The model under review builds one solid part; all positions refer to its coordinate system, in mm. Give positions to 0.01 mm unless a question says otherwise; leave off trailing zeros. Order: outer loops, then holes, each group sorted by start corner. A loop starts at its lowest first (then second) coordinate and runs counter-clockwise, first axis right, second up. Notation, with made-up numbers: M 19.5,26.5 L 62.5,26.5 A16 ccw 62.5,44.5 Z; hole C 17.25,73 d2. An arc over 180 degrees is marked long. One line per question, with ' | ' between items. Start each with the question number.
1. We need section A-A on z = 119. Write out the cut boundary in (x, y), then the cut area to 3 significant figures.
2. Insertion check: P1, Ø2.5, axis at x = 0, z = 342.4, coming from the -Y side; P2, Ø9, axis at x = 0, z = 342.4, coming from the -Y side; P3, Ø9, axis at x = 0, z = 190, coming from the +Y side. Each pin has a flat end and moves straight along its axis. Give the tip position at first contact, or say it passes through.
3. We need section B-B on y = -3.75. Write out the cut boundary in (x, z).
4. Wall thickness on L1, parallel to Y at x = 3.25, z = 20; L2, parallel to X at y = 7.2, z = 240.8: over which ranges is each line inside the solid? List them lowest first.
Autodesk Inventor part; units mm, degrees
ref_plane "YZ Plane" through (0, 0, 0) normal (1, 0, 0) x (0, 1, 0)
ref_plane "XZ Plane" through (0, 0, 0) normal (0, 1, 0) x (-1, 0, 0)
ref_plane "XY Plane" through (0, 0, 0) normal (0, 0, 1) x (1, 0, 0)
sketch "Náčrt1" plane through (0, 0, 0) normal (0, 0, 1) x (1, 0, 0)
  line L0 (-7.5, -7.5) -> (7.5, -7.5)
  line L1 (7.5, -7.5) -> (7.5, 7.5)
  line L2 (7.5, 7.5) -> (-7.5, 7.5)
  line L3 (-7.5, 7.5) -> (-7.5, -7.5)
  line L4 (-7.5, -7.5) -> (7.5, 7.5) construction
  line L5 (7.5, -7.5) -> (-7.5, 7.5) construction
  line L6 (-6.5, -6.5) -> (6.5, -6.5)
  line L7 (6.5, -6.5) -> (6.5, 6.5)
  line L8 (6.5, 6.5) -> (-6.5, 6.5)
  line L9 (-6.5, 6.5) -> (-6.5, -6.5)
  line L10 (-6.5, -6.5) -> (6.5, 6.5) construction
  line L11 (6.5, -6.5) -> (-6.5, 6.5) construction
  point P0 (0, 0)
  dimension "d0" = 15
  dimension "d1" = 15
  dimension "d2" = 13
  dimension "d3" = 13
extrude "Vysunutí1" add sketch "Náčrt1" along normal blind 380
sketch "Náčrt2" plane through (-7.5, 7.5, 0) normal (0, 1, 0) x (1, 0, 0)
  circle A0 centre (7.5, -37.6) radius 1.5
  line L0 (15, 0) -> (0, 0)
  line L1 (0, 0) -> (0, -380)
  line L2 (15, -380) -> (0, -380)
  line L3 (15, 0) -> (15, -380)
  point P0 (7.5, 0)
  dimension "d8" = 3
  dimension "d13" = 37.6
  dimension "d19" = 7.5
extrude "Vysunutí2" cut sketch "Náčrt2" against normal up to surface (1 mm away) contours A0
sketch "Náčrt3" plane through (-7.5, -7.5, 0) normal (0, -1, 0) x (1, 0, 0)
  line L0 (15, 0) -> (0, 0)
  line L1 (0, 0) -> (0, 380)
  line L2 (15, 380) -> (0, 380)
  line L3 (15, 0) -> (15, 380)
  circle A0 centre (7.5, 37.6) radius 1.5
  circle A1 centre (7.5, 37.6) radius 5
  point P0 (7.5, 0)
  dimension "d15" = 10
extrude "Vysunutí3" cut sketch "Náčrt3" against normal up to surface (1 mm away) contours A0 | A1
pattern_linear "Obdélníkové pole1" count 7 spacing 50.8 along (0, 0, 1) of "Vysunutí2"
pattern_linear "Obdélníkové pole2" count 7 spacing 50.8 along (0, 0, 1) of "Vysunutí3"
equation "\"d0\" = width"
equation "\"d1\" = width"
equation "\"d2\" = width - 2 * thickness"
equation "\"d3\" = width - 2 * thickness"
equation "\"d4\" = length"
equation "\"d8\" = HoleDia"
equation "\"d19\" = 0.5 * width"
equation "\"d15\" = HoleDiaOpposite"
equation "\"d22\" = holeDistance"
equation "\"d25\" = holeDistance"
equation "\"width\" = gSquareProfile_Width_Cabinet"
equation "\"thickness\" = gSquareProfile_Thickness_Cabinet"
equation "\"length\" = gCabinet_LogicCircuit_Length - 2 * width"
equation "\"holeDistance\" = 50.8"
equation "\"HoleDiaOpposite\" = 10"
equation "\"HoleDia\" = 3"
properties part number "Profile-Square#07"
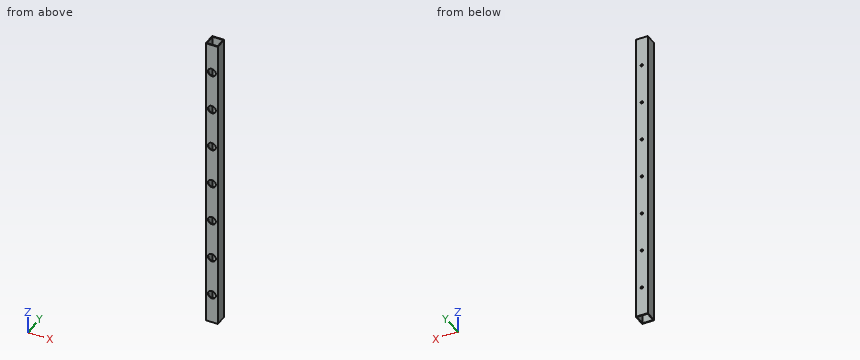
Entries:
1) outline: M -7.5,-7.5 L 7.5,-7.5 L 7.5,7.5 L -7.5,7.5 Z; hole M -6.5,-6.5 L 6.5,-6.5 L 6.5,6.5 L -6.5,6.5 Z | area: 56.0 mm^2
2) P1: passes through | P2: stops at y = 6.5 | P3: stops at y = 7.5
3) outline: M -7.5,0 L -6.5,0 L -6.5,380 L -7.5,380 Z; M 6.5,0 L 7.5,0 L 7.5,380 L 6.5,380 Z
4) L1: y = -7.5 to -6.5, 6.5 to 7.5 | L2: x = -7.5 to -1.5, 1.5 to 7.5
